```python
from build123d import *


with BuildPart() as part:
    # Sketch1 → Revolve1 (revolve)
    with BuildSketch(Plane.XY):
        Polygon((-82.105117767, 11.5), (0, 33.5), (0, 38.5), (-76.4, 18.028681698), (-76.4, 44.496311912), (-102.4, 44.496311912), (-102.4, 41.496311912), (-105.4, 41.496311912), (-105.4, 44.496311912), (-110.4, 44.496311912), (-110.4, 41.496311912), (-113.4, 41.496311912), (-113.4, 44.496311912), (-118.4, 44.496311912), (-118.4, 41.496311912), (-121.4, 41.496311912), (-121.4, 44.496311912), (-126.4, 44.496311912), (-126.4, 36.496311912), (-83.105117767, 11.5), align=None)
    revolve(axis=Axis((0, 0, 0), (-1, 0, 0)))

    # Sketch2 → Cut-Revolve1 (revolve, cut)
    with BuildSketch(Plane.XY):
        Polygon((-11.196152423, 0), (-11.196152423, 35.5), (-11.196152423, 56.271944123), (14.531335426, 56.271944123), (14.531335426, 0), align=None)
    revolve(axis=Axis((0, 0, 0), (-1, 0, 0)), mode=Mode.SUBTRACT)


solid = part.part
```
Source: CAD feature listing. Evaluate the final solid. Frame: model axes, mm. A direction names the side the tool comes from. Give positions to 0.01 mm unless a question says otherwise; leave off trailing zeros. Write each loop counter-clockwise with the first axis right and the second up, starting at its lowest first coordinate (ties: lowest second). Pieces come first, ordered by that corner, then holes.
1. Material intervals for line 1 along X through (y, z) = (-39.5, -13.5); line 2 along Y through (x, z) = (-82.65, 0), sorted ascending.
2. First-contact query: pin 1 (20.5 mm diameter, centred on y = 0, z = 0, fed in from +X); pin 2 (1.5 mm diameter, centred on x = -41.5, y = -10.5, fed in from +Z); pin 3 (3 mm diameter, centred on x = -35, y = -14, fed in from -Z); pin 4 (3 mm diameter, centred on y = -31, z = -32.5, fed in from +X). Flat tips, straight axial feed; report the tip coordinate or a pass-through.
3. Section query B-B (x = -29.5). Return the cut outline in (y, z).
4. Pull-direction query (Y, two-part tool) for faces 3 (the face through (-126.4, -3.5, -36.5)), 4 (the face through (-123.94, -5.79, -44.12)), 5 (the face through (-82.6, -1.5, -11.4)); classes: +Y half, -Y half, draft (parallel to the pull), parting line (faces both ways), or undercut.
5. Section query A-A (x = -70). Return the cut outline in (y, z).
6. Access query for faces 1 (the face through (-110.4, 29.5, 29.5)), 2 (the face through (-115.94, -5.79, -44.12)). Directions: +Z, -Z, +X, -X, +Y, -Y. A direction counts if a zero-diameter tool reaches every point of the face in a straight line with its end or side. Return the directions, or none.
Output values:
1. line 1: x = -126.4 to -121.4, -118.4 to -113.4, -110.4 to -105.4, -102.4 to -76.4
1. line 2: y = -44.5 to -11.5, 11.5 to 44.5
2. pin 1: passes through
2. pin 2: stops at z = 25.66
2. pin 3: stops at z = -26.43
2. pin 4: stops at x = -76.4
3. outline: circle Ø61.19 at (0, 0); hole circle Ø51.19 at (0, 0)
4. face 3: draft
4. face 4: parting line
4. face 5: undercut
5. outline: circle Ø39.49 at (0, 0); hole circle Ø29.49 at (0, 0)
6. face 1: none
6. face 2: +X, -X
